Read the model definition and answer for the solid it produces. Units are mm, in the model's axes. Face numbers are marked on the shaded views. A direction names the side the tool comes from. Round coordinates to 2 decimals unless told otherwise and drop trailing zeros. Write each loop counter-clockwise with the first axis right and the second up, starting at its lowest first coordinate (ties: lowest second). Pieces come first, ordered by that corner, then holes. Notation, with made-up numbers: (-2, 53.25) -> (16, 53.25) arc R36 ccw to (16, 90.25) -> close; hole circle Ø9 at (-12, 28). An arc over 180 degrees is marked (long way). Return JSON: item names as keys, results as strings. Group by question number.
(1) A cutting plane is placed at D-D on x = 17. Give the vertices of the cut face in (y, z).
(2) Given pin 1 (1.3 mm diameter, centred on x = 2, y = -2, fed in from +Z); pin 2 (1.6 mm diameter, centred on x = 12, z = 1, fed in from +Y), each flat-ended and moving along its own axis, determine where each tip first touches the part or whether it passes through.
(3) A cutting plane is placed at B-B on z = 2.75. Give the vertices of the cut face in (x, y).
(4) For the marked faces 4 and 5, determine the directions among +Z, -Z, +X, -X, +Y, -Y from which every point of the face is accessible in a straight line to the end or side of a thin tool.
(5) Straight lines are drawn through the part: line 1 (Y direction, x = 23, z = 1.7); line 2 (X direction, y = -9.25, z = 2.8); line 3 (Y direction, x = 23.75, z = 2.3). For each, find the intervals that lie inside material, in ascending order.
(6) The mould has two halves that part along X. Classify the marked faces 1, 2 and 3: released by +X, released by -X, zero draft, split by the parting line, or undercut.
(7) A cutting plane is placed at C-C on y = -4.5. Give the vertices of the cut face in (x, z), then the cut area to 3 significant figures.
(8) A cutting plane is placed at A-A on y = -14.5. Give the vertices of the cut face in (x, z), then the cut area to 3 significant figures.
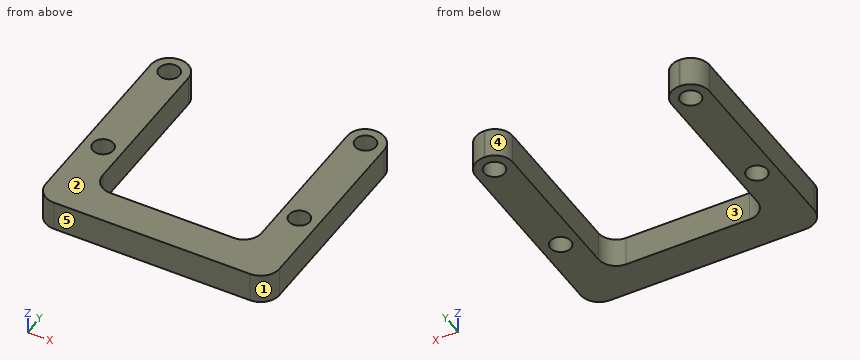
```python
from build123d import *

# Parameters (mm, degrees)
PAD_DEPTH    = 3.2
FILLET_R     = 2
FILLET001_R  = 1.9
SKETCH001_R  = 1.1
POCKET_DEPTH = 5


with BuildPart() as part:
    # Sketch → Pad (new body)
    with BuildSketch(Plane.XY):
        Polygon((0, 0), (4, 0), (4, -20), (21, -20), (21, 0), (25, 0), (25, -23.8), (0, -23.8), align=None)
    extrude(amount=PAD_DEPTH)

    # Fillet
    fillet_edges = [part.edges().sort_by_distance(p)[0] for p in [
        (0, -23.8, 1.6),
        (25, -23.8, 1.6),
        (0, 0, 1.6),
        (25, 0, 1.6),
    ]]
    fillet(fillet_edges, radius=FILLET_R)

    # Fillet001
    fillet001_edges = [part.edges().sort_by_distance(p)[0] for p in [
        (4, 0, 1.6),
        (4, -20, 1.6),
        (21, 0, 1.6),
        (21, -20, 1.6),
    ]]
    fillet(fillet001_edges, radius=FILLET001_R)

    # Sketch001 (on Face5 of Fillet001) → Pocket (cut)
    with BuildSketch(Plane.XY.offset(3.2)):
        with Locations((2, -2)):
            Circle(SKETCH001_R)
        with Locations((2, -14.5)):
            Circle(SKETCH001_R)
        with Locations((23, -2)):
            Circle(SKETCH001_R)
        with Locations((23, -14.5)):
            Circle(SKETCH001_R)
    extrude(amount=-POCKET_DEPTH, mode=Mode.SUBTRACT)


solid = part.part
```
Checks:
{
 "1": {"outline": "(-23.8, 0) -> (-20, 0) -> (-20, 3.2) -> (-23.8, 3.2) -> close"},
 "2": {"pin 1": "passes through", "pin 2": "stops at y = -20"},
 "3": {"outline": "(0, -21.8) arc R2 ccw to (2, -23.8) -> (23, -23.8) arc R2 ccw to (25, -21.8) -> (25, -2) arc R2 ccw to (23, 0) -> (22.9, 0) arc R1.9 ccw to (21, -1.9) -> (21, -18.1) arc R1.9 cw to (19.1, -20) -> (5.9, -20) arc R1.9 cw to (4, -18.1) -> (4, -1.9) arc R1.9 ccw to (2.1, 0) -> (2, 0) arc R2 ccw to (0, -2) -> close; hole circle Ø2.2 at (2, -14.5); hole circle Ø2.2 at (2, -2); hole circle Ø2.2 at (23, -14.5); hole circle Ø2.2 at (23, -2)"},
 "4": {"face 4": "+Z, -Z, +Y", "face 5": "+Z, -Z, +X, -X, -Y"},
 "5": {"line 1": "y = -23.8 to -15.6, -13.4 to -3.1, -0.9 to 0", "line 2": "x = 0 to 4, 21 to 25", "line 3": "y = -23.65 to -15.3, -13.7 to -2.8, -1.2 to -0.15"},
 "6": {"face 1": "released by +X", "face 2": "zero draft", "face 3": "undercut"},
 "7": {"outline": "(0, 0) -> (4, 0) -> (4, 3.2) -> (0, 3.2) -> close; (21, 0) -> (25, 0) -> (25, 3.2) -> (21, 3.2) -> close", "area": "25.6 mm^2"},
 "8": {"outline": "(0, 0) -> (0.9, 0) -> (0.9, 3.2) -> (0, 3.2) -> close; (3.1, 0) -> (4, 0) -> (4, 3.2) -> (3.1, 3.2) -> close; (21, 0) -> (21.9, 0) -> (21.9, 3.2) -> (21, 3.2) -> close; (24.1, 0) -> (25, 0) -> (25, 3.2) -> (24.1, 3.2) -> close", "area": "11.5 mm^2"}
}
